Autodesk Inventor part; units mm, degrees
ref_plane "YZ Plane" through (0, 0, 0) normal (1, 0, 0) x (0, 1, 0)
ref_plane "XZ Plane" through (0, 0, 0) normal (0, 1, 0) x (-1, 0, 0)
ref_plane "XY Plane" through (0, 0, 0) normal (0, 0, 1) x (1, 0, 0)
sketch "Sketch3" plane through (0, 0, 0) normal (0, 1, 0) x (-1, 0, 0)
  line L0 (0, 0) -> (-30, 0)
  line L1 (-30, 0) -> (-30, -60)
  line L2 (-30, -60) -> (0, 0)
  dimension "d10" = 30
  dimension "d11" = 60
  dimension "d33" = 67.082
revolve "Revolution4" add sketch "Sketch3" angle 360 about axis through (0, 0, 0) along (1, 0, 0)
sketch "Sketch4" plane through (30, 0, 0) normal (1, 0, 0) x (0, 0, -1)
  point P0 (0, 0)
  point P1 (0, 0)
hole "Hole1" at (30, 0, 0) direction (-1, 0, 0) diameter 41 depth 40.25
shell "Shell2" thickness 2 removed faces 1 at (30, 15.6337, 43.9334)
sketch "Sketch5" plane through (0, 0, 0) normal (0, 0, 1) x (1, 0, 0)
  circle A0 centre (19.9279, 0) radius 1.5
  point P0 (0, 0)
  dimension "d25" = 3
extrude "Extrusion1" add sketch "Sketch5" along normal blind 21.5 and the other way blind 24
sketch "Sketch6" plane through (19.9279, 0, -24) normal (0, 0, -1) x (-1, 0, 0)
  point P0 (19.9279, 0)
  point P1 (0.0492, -0.0436)
hole "Hole2" at (19.8787, -0.0436, -24) direction (0, 0, 1) diameter 4 depth 48.25
properties part number "Penahan tanah" material "Aluminum 6061-AHC"
Design review of the part built by this model. Coordinates are the model's own, in mm. Give positions to 0.01 mm unless a question says otherwise; leave off trailing zeros. Write each loop counter-clockwise with the first axis right and the second up, starting at its lowest first coordinate (ties: lowest second). Pieces come first, ordered by that corner, then holes. Notation, with made-up numbers: M -23.75,10.5 L -13.75,10.5 A20 ccw -13.75,17.5 Z; hole C 62,50 d9. An arc over 180 degrees is marked long. Answer as a JSON object with one key per item and string values. Group by question number.
1) We need section A-A (z = 0). Give the boundary of the cut face in (x, y), and give its area (3 significant figures).
2) We need section B-B (y = 0). Give the boundary of the cut face in (x, z).
3) Mouldability with a two-part tool opening along X and no side actions: class faces 1 (the face through (17.896, -0.304, -21.434)), 2 (the face through (17.896, -0.304, 21.464)), 3 (the face through (11.485, -22.425, 4.98)), 4 (the face through (14.52, 7.38, -23.43)) as released by +X, released by -X, zero draft, split by the parting line, or undercut.
4) Clearance check with flat-ended pins moving along their axes: pin 1 Ø6 at (x, y) = (26, 22.5) entering from +Z; pin 2 Ø3 at (x, y) = (19.88, -0.04) entering from +Z; pin 3 Ø1 at (x, z) = (25.5, -21.5) entering from -Y; pin 4 Ø24.5 at (y, z) = (0, 0) entering from +X. State where each tip first meets the part, or that it passes through.
5) For line 1 along Y through (x, z) = (20, 17); line 2 along Y through (x, z) = (15.5, -1.5); line 3 along Z through (x, y) = (15.75, 10), list the stretches that pass through material, from the lowest coordinate up.
6) We need section D-D (x = 28). Give the boundary of the cut face in (y, z), and give its area (3 significant figures).
7) We need section C-C (x = 16). Give the boundary of the cut face in (y, z), and give its area (3 significant figures).
Answer key:
{
 "1": {"outline": "M 10.25,-20.5 L 30,-60 L 30,-55.53 L 13.49,-22.5 L 30,-22.5 L 30,-20.5 Z; M 10.25,20.5 L 30,20.5 L 30,22.5 L 13.49,22.5 L 30,55.53 L 30,60 Z", "area": "235 mm²"},
 "2": {"outline": "M 10.25,-20.5 L 30,-60 L 30,-55.53 L 13.49,-22.5 L 17.88,-22.5 L 17.88,-20.5 Z; M 10.25,20.5 L 17.88,20.5 L 17.88,22.5 L 13.49,22.5 L 30,55.53 L 30,60 Z; M 21.88,-22.5 L 30,-22.5 L 30,-20.5 L 21.88,-20.5 Z; M 21.88,20.5 L 30,20.5 L 30,22.5 L 21.88,22.5 Z"},
 "3": {"face 1": "undercut", "face 2": "undercut", "face 3": "released by -X", "face 4": "released by +X"},
 "4": {"pin 1": "stops at z = 53.58", "pin 2": "stops at z = 42.76", "pin 3": "stops at y = -47.37", "pin 4": "passes through"},
 "5": {"line 1": "y = -36.21 to -31.2, -14.74 to -11.46, 11.46 to 14.74, 31.2 to 36.21", "line 2": "y = -30.96 to -26.49, -22.45 to -20.45, 20.45 to 22.45, 26.49 to 30.96", "line 3": "z = -29.87 to -25.11, -20.16 to -17.9, 17.9 to 20.16, 25.11 to 29.87"},
 "6": {"outline": "C 0,0 d112; C 0,0 d45; hole C 0,0 d103.06; hole C 0,0 d41", "area": "1,780 mm²"},
 "7": {"outline": "C 0,0 d64; C 0,0 d45; hole C 0,0 d55.06; hole C 0,0 d41", "area": "1,110 mm²"}
}
